Geometry: final body of the model. Coordinates: model frame, mm. Face numbers are marked on the shaded views. Coordinates: 2 decimals unless noted, no trailing zeros. Loops run counter-clockwise (first coordinate to the right, second up) from the corner with the lowest first, then second, coordinate; pieces in that order, holes last. Notation, with made-up numbers: (86.25, 62.25) -> (114.25, 62.25) arc R15 cw to (114.25, 75.25) -> close; hole circle Ø9 at (76.25, 59). An arc over 180 degrees is marked (long way). One line per item, written item: value. Start each with the question number.
Item 1: Ray query, probe 1 along Z at (x, y) = (-4.5, -5); probe 2 along Z at (x, y) = (4, -3.75); probe 3 along X at (y, z) = (-4, -4.75). Return the intervals inside material, ascending. Write a range as from..to.
Item 2: Section query B-B on z = 0. Return loops of the section in (x, y).
Item 3: Contact query for flat-ended pins moving along their axis: pin 1 Ø1 at (y, z) = (-5.5, 1.5) entering from +X; pin 2 Ø4 at (y, z) = (-6.5, -5.5) entering from -X; pin 3 Ø1.5 at (x, z) = (2.5, -1) entering from +Y. Output: stop coordinate, or through.
Item 4: Section query D-D on y = -7.25. Return loops of the section in (x, z).
Item 5: Mould query, pull axis Y, two halves, no side actions, for the marked faces 1, 2 and 3. Classes: +Y half, -Y half, draft (parallel to the pull), parting line (faces both ways), or undercut.
Item 6: Section query A-A on x = 0. Return loops of the section in (y, z), then the cut area to 3 significant figures.
Item 7: Section query C-C on y = -5.75. Return loops of the section in (x, z).
from build123d import *


with BuildPart() as part:
    # Sketch1 → Revolve1 (revolve)
    with BuildSketch(Plane.XY):
        with BuildLine():
            Line((-7.990929537, -3.644388375), (-8.41, -9.96))
            Line((-8.41, -9.96), (-6.89, -9.96))
            Line((-6.89, -9.96), (-6.79, -9.96))
            Line((-6.79, -9.96), (-6.79, -9.46))
            Line((-6.79, -9.46), (-7.29, -9.46))
            Line((-7.29, -9.46), (-6.934045173, -4.095574106))
            ThreePointArc((-6.934045173, -4.095574106), (-6.919243429, -4.038745871), (-6.884556501, -3.991360674))
            ThreePointArc((-6.884556501, -3.991360674), (-3.699614673, -1.98226408), (0, -1.28))
            Line((0, -1.28), (0, 0))
            ThreePointArc((0, 0), (-4.111446691, -0.768945317), (-7.667085246, -2.971830982))
            ThreePointArc((-7.667085246, -2.971830982), (-7.894114775, -3.276759708), (-7.990929537, -3.644388375))
        make_face()
    revolve(axis=Axis((0, 0, 0), (0, 1, 0)))


solid = part.part
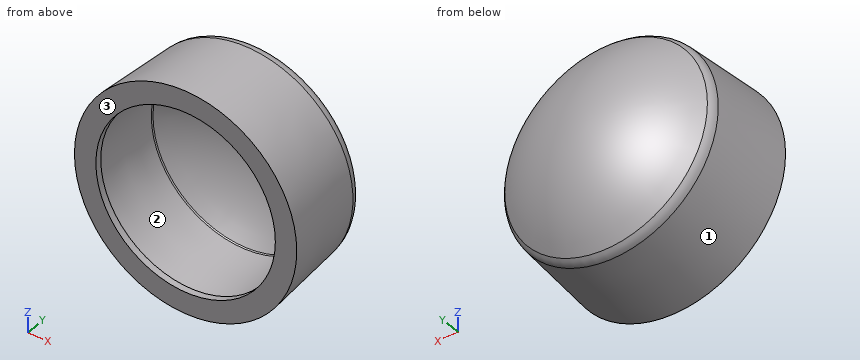
Reply:
1. probe 1: z = -6.71..-5.35, 5.35..6.71
1. probe 2: z = -6.93..-5.27, 5.27..6.93
1. probe 3: x = -6.46..-5, 5..6.46
2. outline: (-8.41, -9.96) -> (-6.79, -9.96) -> (-6.79, -9.46) -> (-7.29, -9.46) -> (-6.93, -4.1) arc R0.16 cw to (-6.88, -3.99) arc R10.1 cw to (6.88, -3.99) arc R0.16 cw to (6.93, -4.1) -> (7.29, -9.46) -> (6.79, -9.46) -> (6.79, -9.96) -> (8.41, -9.96) -> (7.99, -3.64) arc R1 ccw to (7.67, -2.97) arc R11.38 ccw to (-7.67, -2.97) arc R1 ccw to (-7.99, -3.64) -> close
3. pin 1: stops at x = 8.06
3. pin 2: stops at x = -7.41
3. pin 3: stops at y = -0.17
4. outline: circle Ø16.46 at (0, 0); hole circle Ø14.29 at (0, 0)
5. face 1: +Y half
5. face 2: undercut
5. face 3: -Y half
6. outline: (-9.96, -8.41) -> (-3.64, -7.99) arc R1 ccw to (-2.97, -7.67) arc R11.38 ccw to (-2.97, 7.67) arc R1 ccw to (-3.64, 7.99) -> (-9.96, 8.41) -> (-9.96, 6.79) -> (-9.46, 6.79) -> (-9.46, 7.29) -> (-4.1, 6.93) arc R0.16 cw to (-3.99, 6.88) arc R10.1 cw to (-3.99, -6.88) arc R0.16 cw to (-4.1, -6.93) -> (-9.46, -7.29) -> (-9.46, -6.79) -> (-9.96, -6.79) -> close
6. area: 35.3 mm²
7. outline: circle Ø16.26 at (0, 0); hole circle Ø14.09 at (0, 0)
